Check sheet for the modelled part. Datum: model origin and axes. Units: mm. A direction names the side the tool comes from. Round coordinates to 2 decimals unless told otherwise and drop trailing zeros. Order: outer loops, then holes, each group sorted by start corner. A loop starts at its lowest first (then second) coordinate and runs counter-clockwise, first axis right, second up.
Q1. Scan lines: probe 1 along X at (y, z) = (-0.9, 0); probe 2 along Z at (x, y) = (0, -1.85); probe 3 along X at (y, z) = (29.5, 20). Record each from-to range of solid material in increasing order.
Q2. Depth check by flat-ended pin: P1, Ø2.5, axis at x = 0, z = 0, coming from the +Y side; P2, Ø6.5, axis at x = 0, z = 77, coming from the +Y side; P3, Ø4, axis at x = -8, z = 21, coming from the +Y side. Enter the tip coordinate at first touch or a pass-through.
Q3. Set-up check for faces 1 (the flat face through (132, 21, 39)), 2 (the flat face through (-11, 14, 39)), 3 (the flat face through (-10.93, 39.874, 21.92)), 4 (the flat face through (3.456, -2, 38)): record each of +Z, -Z, +X, -X, +Y, -Y from which the full face is reachable in a straight line by a thin tool's end or side.
Q4. Cross-section at B-B on x = 126. Record the cut outline in (y, z).
Q5. Cross-section at C-C on z = 19.5. Record the cut outline in (x, y).
Q6. Mould release check, pull along Y, two halves, no side actions. Record for faces 5 (the flat face through (135.27, 50.04, 33.92)), 6 (the flat face through (136.93, 38.773, 21.149)), 7 (the flat face through (64, -2, -0.906)): +Y half, -Y half, draft (parallel to the pull), parting line (faces both ways), or undercut.
Q7. Cross-section at D-D on y = 36.5. Give the number of separate pieces and of enclosed holes in the cut face, then the cut area to 3 significant figures.
Q8. Cross-section at A-A on x = 22. Record the cut outline in (y, z).
Autodesk Fusion 360 part; units mm, degrees
sketch "Sketch2" plane through (0, 0, 0) normal (0, 1, 0) x (1, 0, 0)
  line L0 (0, 0) -> (126, 0) construction
  line L1 (0, 0) -> (0, -77) construction
  circle A0 centre (126, 0) radius 2
  circle A1 centre (0, 0) radius 2
  circle A2 centre (0, -77) radius 2
  line L2 (126, 0) -> (126, -77) construction
  circle A3 centre (126, -77) radius 2
  line L3 (3.4555, -78.0942) -> (122.9555, -78.0942)
  line L4 (122.9555, -78.0942) -> (122.9555, 0.9058)
  line L5 (122.9555, 0.9058) -> (3.4555, 0.9058)
  line L6 (3.4555, 0.9058) -> (3.4555, -78.0942)
  line L7 (-6, -77) -> (-6, -83) construction
  line L8 (-6, -83) -> (0, -83) construction
  line L9 (-6, -83) -> (132, -83)
  line L10 (132, -83) -> (132, 6)
  line L11 (132, 6) -> (-6, 6)
  line L12 (-6, 6) -> (-6, -83)
  dimension "d16" = 4
  dimension "d17" = 4
  dimension "d18" = 4
  dimension "d20" = 4
  dimension "d23" = 6
  dimension "d24" = 6
  dimension "d25" = 138
  dimension "d26" = 89
extrude "Extrude2" add sketch "Sketch2" against normal blind 3.5
sketch "Sketch3" plane through (132, 0, 0) normal (1, 0, 0) x (0, 1, 0)
  line L0 (0, -6) -> (0, 83)
  line L1 (0, 83) -> (-3.5, 83)
  line L2 (-3.5, 83) -> (-3.5, -6)
  line L3 (-3.5, -6) -> (0, -6)
  line L4 (0, -6) -> (78.6469, 49.0692)
  line L5 (0, -6) -> (96.0102, -6) construction
  line L6 (78.6469, 49.0692) -> (0, 83)
  dimension "d29" = 35
extrude "Extrude3" add sketch "Sketch3" along normal blind 10
sketch "Sketch4" plane through (-6, 0, 0) normal (-1, 0, 0) x (0, -1, 0)
  line L0 (0, 83) -> (0, -6)
  line L1 (0, -6) -> (3.5, -6)
  line L2 (3.5, -6) -> (3.5, 83)
  line L3 (3.5, 83) -> (0, 83)
  line L4 (0, 83) -> (-78.6469, 49.0692)
  line L5 (-78.6469, 49.0692) -> (0, -6)
  point P0 (-78.6469, 49.0692)
extrude "Extrude4" add sketch "Sketch4" along normal blind 10
sketch "Sketch5" plane through (0, 2.8191, -4.0261) normal (0, 0.5736, -0.8192) x (-1, 0, 0)
  line L0 (-132, -3.4415) -> (-132, 92.5687)
  line L1 (-132, 92.5687) -> (-142, 92.5687)
  line L2 (-142, 92.5687) -> (-142, -3.4415)
  line L3 (-142, -3.4415) -> (-132, -3.4415)
  line L4 (-137, 92.5687) -> (-137, -3.4415) construction
  line L5 (6, 47.6068) -> (-132, 47.6068)
  line L6 (-63, 47.6068) -> (-63, 87.5387) construction
  line L7 (-137, 92.5687) -> (-137, 77.5687) construction
  circle A0 centre (-137, 77.5687) radius 2
  circle A1 centre (-137, 58.7979) radius 2
  circle A2 centre (11, 77.5687) radius 2
  circle A3 centre (11, 58.7979) radius 2
  circle A4 centre (-137, 77.5687) radius 4
  circle A5 centre (-137, 58.7979) radius 4
  circle A6 centre (11, 58.7979) radius 4
  circle A7 centre (11, 77.5687) radius 4
  dimension "d34" = 15
  dimension "d35" = 4
  dimension "d36" = 4
  dimension "d39" = 8
  dimension "d40" = 8
extrude "Extrude6" cut sketch "Sketch5" against normal blind 64 contours A0 | A1 | A2 | A3
ref_plane "WorkPlane1" through (137, 37.0292, 24.8112) normal (0, 0.5736, -0.8192) x (0, 0.8192, 0.5736)
sketch "Sketch6" plane through (137, 37.0292, 24.8112) normal (0, 0.5736, -0.8192) x (0, 0.8192, 0.5736)
  circle A0 centre (33.0958, 0) radius 4
  circle A1 centre (14.1568, -0.0063) radius 4
  line L0 (3.0432, -143) -> (3.0432, -5)
  line L1 (3.0432, -74) -> (11.3701, -74) construction
  circle A2 centre (33.0958, -148) radius 4
  circle A3 centre (14.1568, -147.9937) radius 4
  dimension "d44" = 8
  dimension "d45" = 8
extrude "Extrude7" cut sketch "Sketch6" against normal blind 65
sketch "Sketch7" plane through (-6, 0, 0) normal (1, 0, 0) x (0, 1, 0)
  line L0 (0, 83) -> (0, -6)
  line L1 (0, -6) -> (78.6469, 49.0692)
  line L2 (78.6469, 49.0692) -> (0, 83)
  line L3 (2.5489, 73.8327) -> (2.5489, 2.9392)
  line L4 (2.5489, 2.9392) -> (32.8483, 25.9556)
  line L5 (32.8483, 25.9556) -> (10.651, 69.2676)
  line L6 (10.651, 69.2676) -> (2.5489, 73.8327)
extrude "Extrude8" cut sketch "Sketch7" against normal blind 5 contours L3 L4 L5 L6
Results found:
1. probe 1: x = -16 to -2, 2 to 3.46, 122.96 to 124, 128 to 142
1. probe 2: z = -6 to -2, 2 to 75, 79 to 83
1. probe 3: x = -16 to -6, 132 to 142
2. P1: passes through
2. P2: stops at y = 0
2. P3: stops at y = 41.42
3. face 1: +Z, -Z, +Y
3. face 2: none
3. face 3: -Z, +X, -X, +Y
3. face 4: +Y, -Y
4. outline: (-3.5, -6) - (0, -6) - (0, -2) - (-3.5, -2) - close; (-3.5, 2) - (0, 2) - (0, 75) - (-3.5, 75) - close; (-3.5, 79) - (0, 79) - (0, 83) - (-3.5, 83) - close
5. outline: (-16, -3.5) - (3.46, -3.5) - (3.46, 0) - (-6, 0) - (-6, 2.55) - (-11, 2.55) - (-11, 24.35) - (-6, 24.35) - (-6, 36.42) - (-16, 36.42) - close; (122.96, -3.5) - (142, -3.5) - (142, 36.42) - (132, 36.42) - (132, 0) - (122.96, 0) - close
6. face 5: undercut
6. face 6: +Y half
6. face 7: draft
7. separate pieces: 2
7. enclosed holes: 2
7. area: 779 mm2
8. outline: (-3.5, -6) - (0, -6) - (0, -0.91) - (-3.5, -0.91) - close; (-3.5, 78.09) - (0, 78.09) - (0, 83) - (-3.5, 83) - close
